```python
from build123d import *

# Parameters (mm, degrees)
SKETCH1_R                      = 31.75
BOSS_EXTRUDE1_DEPTH            = 9.525
SKETCH2_R                      = 14
CUT_EXTRUDE1_DEPTH             = 3
F_8_CLEARANCE_HOLE1_D          = 4.3053
SKETCH5_R                      = 12.7
CUT_EXTRUDE2_DEPTH             = 4.7498
SKETCH6_R                      = 6
CUT_EXTRUDE3_DEPTH             = 46.154485215
CBORE_FOR_M4_SHCS1_D           = 4.5
CBORE_FOR_M4_SHCS1_CBORE_D     = 8
CBORE_FOR_M4_SHCS1_CBORE_DEPTH = 4
SKETCH9_OUTSIDE_W              = 83.562
SKETCH9_OUTSIDE_H              = 83.562
SKETCH9_OUTSIDE_R              = 23.749
CUT_EXTRUDE4_DEPTH             = 3.175


with BuildPart() as part:
    # Sketch1 → Boss-Extrude1 (new body)
    with BuildSketch(Plane.XY):
        with Locations(Location((0, 0, 0), (0, 0, 180))):
            Circle(SKETCH1_R)
    extrude(amount=BOSS_EXTRUDE1_DEPTH)

    # Sketch2 → Cut-Extrude1 (cut)
    with BuildSketch(Plane.XY.offset(9.525)):
        Circle(SKETCH2_R)
    extrude(amount=-CUT_EXTRUDE1_DEPTH, mode=Mode.SUBTRACT)

    # #8 Clearance Hole1 (through all)
    with Locations(Plane.XY.offset(9.525)):
        with Locations((0, 28.575), (24.746675913, 14.2875), (24.746675913, -14.2875), (0, -28.575), (-24.746675913, -14.2875), (-24.746675913, 14.2875)):
            Hole(F_8_CLEARANCE_HOLE1_D / 2)

    # Sketch5 → Cut-Extrude2 (cut)
    with BuildSketch(Plane(origin=(0, 0, 0), x_dir=(-1, 0, 0), z_dir=(0, 0, -1))):
        Circle(SKETCH5_R)
    extrude(amount=-CUT_EXTRUDE2_DEPTH, mode=Mode.SUBTRACT)

    # Sketch6 → Cut-Extrude3 (cut, through all)
    with BuildSketch(Plane(origin=(0, 0, 4.7498), x_dir=(-1, 0, 0), z_dir=(0, 0, -1))):
        Circle(SKETCH6_R)
    extrude(amount=-CUT_EXTRUDE3_DEPTH, mode=Mode.SUBTRACT)

    # CBORE for M4 SHCS1 (through all)
    with Locations(Plane(origin=(0, 0, 0), x_dir=(-1, 0, 0), z_dir=(0, 0, -1))):
        with Locations((0, 17.5), (17.5, 0), (0, -17.5), (-17.5, 0)):
            CounterBoreHole(CBORE_FOR_M4_SHCS1_D / 2, CBORE_FOR_M4_SHCS1_CBORE_D / 2, CBORE_FOR_M4_SHCS1_CBORE_DEPTH)

    # Sketch9 outside → Cut-Extrude4 (cut)
    with BuildSketch(Plane.XY.offset(9.525)):
        Rectangle(SKETCH9_OUTSIDE_W, SKETCH9_OUTSIDE_H)
        Circle(SKETCH9_OUTSIDE_R, mode=Mode.SUBTRACT)
    extrude(amount=-CUT_EXTRUDE4_DEPTH, mode=Mode.SUBTRACT)


solid = part.part
```
Input: part model. Units: mm. Frame: model coordinates. A direction names the side the tool comes from. Coordinates: 2 decimals unless noted, no trailing zeros. Write each loop counter-clockwise with the first axis right and the second up, starting at its lowest first coordinate (ties: lowest second). Pieces come first, ordered by that corner, then holes. Notation, with made-up numbers: (-9, 21) -> (18, 21) arc R21 cw to (18, 38) -> close; hole circle Ø5 at (61, 18.25). An arc over 180 degrees is marked (long way). Write each question's results on one line, items separated by ' | '.
Item 1: Section query B-B on y = 11. Return loops of the section in (x, z) (3 decimals).
Conclusion:
outline: (-29.784, 0) -> (-6.347, 0) -> (-6.347, 4.75) -> (6.347, 4.75) -> (6.347, 0) -> (29.784, 0) -> (29.784, 6.35) -> (21.048, 6.35) -> (21.048, 9.525) -> (8.66, 9.525) -> (8.66, 6.525) -> (-8.66, 6.525) -> (-8.66, 9.525) -> (-21.048, 9.525) -> (-21.048, 6.35) -> (-29.784, 6.35) -> close
Item 2: Section query C-C on x = -24.5. Return loops of the section in (y, z).
Conclusion:
outline: (-20.19, 0) -> (-16.43, 0) -> (-16.43, 6.35) -> (-20.19, 6.35) -> close; (-12.15, 0) -> (12.15, 0) -> (12.15, 6.35) -> (-12.15, 6.35) -> close; (16.43, 0) -> (20.19, 0) -> (20.19, 6.35) -> (16.43, 6.35) -> close
Item 3: Section query A-A on x = 17.5. Return loops of the section in (y, z) (3 decimals).
Conclusion:
outline: (-26.492, 0) -> (-4, 0) -> (-4, 4) -> (-2.25, 4) -> (-2.25, 9.525) -> (-16.055, 9.525) -> (-16.055, 6.35) -> (-26.492, 6.35) -> close; (2.25, 4) -> (4, 4) -> (4, 0) -> (26.492, 0) -> (26.492, 6.35) -> (16.055, 6.35) -> (16.055, 9.525) -> (2.25, 9.525) -> close
Item 4: Mould query, pull axis Y, two halves, no side actions, for faces 4 (the cylindrical face through (22.652, 7.134, 7.96)), 5 (the flat face through (2, 24, 6.35)), 6 (the flat face through (-2, -19, 4)). Classes: +Y half, -Y half, draft (parallel to the pull), parting line (faces both ways), or undercut.
Conclusion:
face 4: parting line | face 5: draft | face 6: undercut
Item 5: Section query D-D on z = 1.5. Count the separate pieces of the cut face and the enclosed holes in it, plus the area to 3 significant figures.
Conclusion:
separate pieces: 1 | enclosed holes: 11 | area: 2,370 mm^2
Item 6: Pin query (flat end, axial travel): pin 1 Ø2 at (x, z) = (5, 8) entering from +Y; pin 2 Ø2.5 at (x, y) = (18, 1) entering from -Z; pin 3 Ø5 at (x, y) = (0, -28.575) entering from +Z. Return the tip coordinate at first contact, or that it passes through.
Conclusion:
pin 1: stops at y = 23.41 | pin 2: stops at z = 4 | pin 3: stops at z = 6.35
Item 7: Set-up query: faces 1 (the cylindrical face through (-15.354, 0.676, 6.801)), 2 (the cylindrical face through (12.932, -5.362, 8.046)), 3 (the flat face through (-2, 16, 4)). Return all of +Z, -Z, +X, -X, +Y, -Y with unobstructed straight access to the full face (end or side cutting, diameter ignored); none if empty.
Conclusion:
face 1: +Z, -Z | face 2: +Z | face 3: -Z
Item 8: Material intervals for probe 1 along Y at (x, z) = (0, 3.2); probe 2 along X at (y, z) = (-13, 5.5); probe 3 along Y at (x, z) = (26, 4), sorted ascending.
Conclusion:
probe 1: y = -31.75 to -30.73, -26.42 to -21.5, -13.5 to -12.7, 12.7 to 13.5, 21.5 to 26.42, 30.73 to 31.75 | probe 2: x = -28.97 to -26.47, -23.02 to 23.02, 26.47 to 28.97 | probe 3: y = -18.22 to -16.04, -12.54 to 12.54, 16.04 to 18.22
